Autodesk Inventor part; units mm, degrees
ref_plane "YZ Plane" through (0, 0, 0) normal (1, 0, 0) x (0, 1, 0)
ref_plane "XZ Plane" through (0, 0, 0) normal (0, 1, 0) x (-1, 0, 0)
ref_plane "XY Plane" through (0, 0, 0) normal (0, 0, 1) x (1, 0, 0)
sketch "Sketch1" plane through (0, 0, 0) normal (0, 1, 0) x (-1, 0, 0)
  line L0 (5, 95.202) -> (-5, 95.202)
  line L1 (-5, 95.202) -> (-5, -95.202)
  line L2 (-5, -95.202) -> (5, -95.202)
  line L3 (5, -95.202) -> (5, 95.202)
  line L4 (5, 95.202) -> (-5, -95.202) construction
  line L5 (-5, 95.202) -> (5, -95.202) construction
  line L6 (3, 101.655) -> (-3, 101.655)
  line L7 (-3, 101.655) -> (-3, -101.655)
  line L8 (-3, -101.655) -> (3, -101.655)
  line L9 (3, -101.655) -> (3, 101.655)
  line L10 (3, 101.655) -> (-3, -101.655) construction
  line L11 (-3, 101.655) -> (3, -101.655) construction
  line L12 (-3, -13) -> (3, -13)
  line L13 (3, -13) -> (3, -7)
  line L14 (3, -7) -> (-3, -7)
  line L15 (-3, -7) -> (-3, -13)
  line L16 (-3, -15) -> (3, -15)
  line L17 (3, -5) -> (-3, -5)
  point P0 (0, 0)
  point P1 (0, -7)
  point P2 (-3, -95.202)
  point P3 (3, -95.202)
  point P4 (3, 95.202)
  point P5 (-3, 95.202)
  point P6 (-3, -7)
  dimension "d0" = 10
  dimension "d1" = 190.404
  dimension "d2" = 203.31
  dimension "d4" = 6
  dimension "d5" = 82.202
  dimension "d6" = 6
  dimension "d7" = 6
  dimension "d8" = 2
  dimension "d9" = 2
extrude "Extrusion1" add sketch "Sketch1" along normal blind 75
extrude "Extrusion2" add sketch "Sketch1" against normal blind 20 contours L9 L17 L7 L0 | L2 L7 L16 L9 | L9 L12 L7 L14
sketch "Sketch2" plane through (5, 0, 95.202) normal (1, 0, 0) x (0, 0, -1)
  circle A0 centre (20, 12) radius 7.5
  line L0 (0, 0) -> (0, 75)
  line L1 (0, 0) -> (190.404, 0)
  point P0 (95.202, 0)
  dimension "d14" = 15
  dimension "d15" = 20
  dimension "d16" = 12
extrude "Extrusion3" cut sketch "Sketch2" against normal blind 75
sketch "Sketch3" plane through (0, 75, 0) normal (0, 1, 0) x (1, 0, 0)
  line L0 (-3, -101.655) -> (3, -101.655)
  line L1 (-5, 95.202) -> (-5, -95.202)
  point P0 (0, 0)
  point P1 (0, 0)
  dimension "d26" = 101.655
  dimension "d27" = 5
hole "Hole1" at (0, 75, 0) direction (0, -1, 0) diameter 4 depth 7 countersink diameter 4.2 countersink angle 90
sketch "Sketch4" plane through (0, -20, 0) normal (0, -1, 0) x (1, 0, 0)
  line L0 (3, -13) -> (3, -7)
  point P0 (0, 0)
  point P1 (0, -9.8779)
  dimension "d28" = 3
hole "Hole2" at (0, -20, -9.8779) direction (0, 1, 0) diameter 4 depth 7 countersink diameter 4.2 countersink angle 90
properties part number "sciana_dluga" material "ABS Plastic"
The model under review builds one solid part; all positions refer to its coordinate system, in mm. A direction names the side the tool comes from. Round coordinates to 2 decimals unless told otherwise and drop trailing zeros. Order: outer loops, then holes, each group sorted by start corner. A loop starts at its lowest first (then second) coordinate and runs counter-clockwise, first axis right, second up. Notation, with made-up numbers: (-13, 74.25) -> (11, 74.25) arc R20 cw to (11, 90.25) -> close; hole circle Ø8 at (74, 22.25). An arc over 180 degrees is marked (long way). Use a Markdown table: item, result.
Q1. For line 1 (Z direction, x = 0, y = -15); line 2 (Z direction, x = 0, y = 71.75) (3 decimals); line 3 (Y direction, x = 4, z = -58), list the stretches that pass through material, from the lowest coordinate up.
Values:
| item | result |
|---|---|
| line 1 | z = -95.2 to -15, -13 to -11.88, -7.88 to -7, -5 to 95.2 |
| line 2 | z = -101.655 to -2, 2 to 101.655 |
| line 3 | y = 0 to 75 |
Q2. We need section A-A on y = 12. Write out the cut boundary in (x, z) (3 decimals).
Values:
| item | result |
|---|---|
| outline | (-5, -95.202) -> (-3, -95.202) -> (-3, -101.655) -> (3, -101.655) -> (3, -95.202) -> (5, -95.202) -> (5, 67.702) -> (-5, 67.702) -> close; (-5, 82.702) -> (5, 82.702) -> (5, 95.202) -> (3, 95.202) -> (3, 101.655) -> (-3, 101.655) -> (-3, 95.202) -> (-5, 95.202) -> close |
Q3. We need section C-C on z = 52.5. Write out the cut boundary in (x, y).
Values:
| item | result |
|---|---|
| outline | (-5, 0) -> (-3, 0) -> (-3, -20) -> (3, -20) -> (3, 0) -> (5, 0) -> (5, 75) -> (-5, 75) -> close |
Q4. Clearance check with flat-ended pins moving along their axes: P1, Ø1.2, axis at x = -1, z = -9, coming from the -Y side; P2, Ø3, axis at x = 1, y = -12, coming from the +Z side; P3, Ø5, axis at y = -10.5, z = -8.5, coming from the -X side. State where each tip first meets the part, or that it passes through.
Values:
| item | result |
|---|---|
| P1 | stops at y = -13 |
| P2 | stops at z = 95.2 |
| P3 | stops at x = -3 |
Q5. We need section D-D on z = 0. Write out the cut boundary in (x, y).
Values:
| item | result |
|---|---|
| outline | (-5, 0) -> (-3, 0) -> (-3, -20) -> (3, -20) -> (3, 0) -> (5, 0) -> (5, 75) -> (2.1, 75) -> (2, 74.9) -> (2, 68) -> (-2, 68) -> (-2, 74.9) -> (-2.1, 75) -> (-5, 75) -> close |
Q6. Mouldability with a two-part tool opening along Z and no side actions: class faces 4 (the flat face through (-3, 37, -98)), 5 (the cylindrical face through (0.07, 12.33, 82.695)), 6 (the flat face through (0, -10, 95.202)) as +Z half, -Z half, draft (parallel to the pull), parting line (faces both ways), or undercut.
Values:
| item | result |
|---|---|
| face 4 | draft |
| face 5 | undercut |
| face 6 | +Z half |
Q7. Tool access review of faces 1 (the flat face through (-3, -10, -10)), 2 (the flat face through (3, 37, -98)), 3 (the flat face through (0, -10, -13)): name each direction out of +Z, -Z, +X, -X, +Y, -Y from which nothing blocks a thin tool from reaching the whole face with its end or side.
Values:
| item | result |
|---|---|
| face 1 | +Z, -Z, -X, -Y |
| face 2 | -Z, +X, +Y, -Y |
| face 3 | +X, -X, -Y |
